```python
from build123d import *

# Parameters (mm, degrees)
SKETCH1_R           = 19.05
BOSS_EXTRUDE1_DEPTH = 1.5875
SKETCH2_R           = 17.4625
BOSS_EXTRUDE2_DEPTH = 12.7
SKETCH3_R           = 7.9375
CUT_EXTRUDE1_DEPTH  = 15.2875
FILLET1_R           = 0.254


with BuildPart() as part:
    # Sketch1 → Boss-Extrude1 (new body)
    with BuildSketch(Plane(origin=(0, 0, 0), x_dir=(1, 0, 0), z_dir=(0, 1, 0))):
        Circle(SKETCH1_R)
    extrude(amount=BOSS_EXTRUDE1_DEPTH)

    # Sketch2 → Boss-Extrude2 (add)
    with BuildSketch(Plane(origin=(0, 1.5875, 0), x_dir=(1, 0, 0), z_dir=(0, 1, 0))):
        Circle(SKETCH2_R)
    extrude(amount=BOSS_EXTRUDE2_DEPTH)

    # Sketch3 → Cut-Extrude1 (cut, through all)
    with BuildSketch(Plane(origin=(0, 14.2875, 0), x_dir=(1, 0, 0), z_dir=(0, 1, 0))):
        Circle(SKETCH3_R)
    extrude(amount=-CUT_EXTRUDE1_DEPTH, mode=Mode.SUBTRACT)

    # Fillet1
    fillet1_edges = [part.edges().sort_by_distance(p)[0] for p in [
        (-7.9375, 14.2875, 0),
        (-19.05, 0, 0),
        (-19.05, 1.5875, 0),
        (-17.4625, 14.2875, 0),
    ]]
    fillet(fillet1_edges, radius=FILLET1_R)


solid = part.part
```
The model under review builds one solid part; all positions refer to its coordinate system, in mm. A direction names the side the tool comes from. Round coordinates to 2 decimals unless told otherwise and drop trailing zeros. Loops run counter-clockwise (first coordinate to the right, second up) from the corner with the lowest first, then second, coordinate; pieces in that order, holes last. Notation, with made-up numbers: M 9.5,33.25 L 43.5,33.25 A19 ccw 43.5,69.25 Z; hole C 5,38 d8. An arc over 180 degrees is marked long. Answer as a JSON object with one key per item and string values.
(1) To check wall thickness, follow line 1 along Z through (x, y) = (0, 8.75); line 2 along X through (y, z) = (6.75, -6.5). State the ranges of each line that lie inside material, in increasing order.
Resolved:
{"line 1": "-17.46 to -7.94, 7.94 to 17.46", "line 2": "-16.21 to -4.56, 4.56 to 16.21"}
(2) Take a section at C-C on y = 10.5. Give the boundary of the cut face in (x, z) (1 decimal), and give its area (3 significant figures).
Resolved:
{"outline": "C 0,0 d34.9; hole C 0,0 d15.9", "area": "760 mm²"}
(3) Draft analysis for pull direction Z (two halves, no side actions). For faces 1 (the flat face through (8.1, 0, -0.3)), 2 (the cylindrical face through (-15.12, 0.79, 11.59)), 3 (the cylindrical face through (-1.72, 7.11, 7.75)), state which applies: released by +Z, released by -Z, zero draft, split by the parting line, or undercut.
Resolved:
{"face 1": "zero draft", "face 2": "split by the parting line", "face 3": "undercut"}
(4) Take a section at A-A on x = 0. Give the boundary of the cut face in (y, z).
Resolved:
{"outline": "M 0,-18.8 A0.25 ccw 0.25,-19.05 L 1.33,-19.05 A0.25 ccw 1.59,-18.8 L 1.59,-17.46 L 14.03,-17.46 A0.25 ccw 14.29,-17.21 L 14.29,-8.19 A0.25 ccw 14.03,-7.94 L 0,-7.94 Z; M 0,7.94 L 14.03,7.94 A0.25 ccw 14.29,8.19 L 14.29,17.21 A0.25 ccw 14.03,17.46 L 1.59,17.46 L 1.59,18.8 A0.25 ccw 1.33,19.05 L 0.25,19.05 A0.25 ccw 0,18.8 Z"}
(5) Tool access review of faces 4 (the flat face through (7.4, 14.288, -4.1)), 5 (the flat face through (5, 1.588, 17)): name each direction out of +Z, -Z, +X, -X, +Y, -Y from which nothing blocks a thin tool from reaching the whole face with its end or side.
Resolved:
{"face 4": "+Z, -Z, +X, -X, +Y", "face 5": "+Y"}
(6) Take a section at B-B on z = 0. Give the boundary of the cut face in (x, y), and give its area (3 significant figures).
Resolved:
{"outline": "M -19.05,0.25 A0.25 ccw -18.8,0 L -7.94,0 L -7.94,14.03 A0.25 ccw -8.19,14.29 L -17.21,14.29 A0.25 ccw -17.46,14.03 L -17.46,1.59 L -18.8,1.59 A0.25 ccw -19.05,1.33 Z; M 7.94,0 L 18.8,0 A0.25 ccw 19.05,0.25 L 19.05,1.33 A0.25 ccw 18.8,1.59 L 17.46,1.59 L 17.46,14.03 A0.25 ccw 17.21,14.29 L 8.19,14.29 A0.25 ccw 7.94,14.03 Z", "area": "277 mm²"}
(7) Clearance check with flat-ended pins moving along their axes: P1, Ø1, axis at x = 4.5, y = 7, coming from the -Z side; P2, Ø4, axis at x = 7.5, y = 8, coming from the +Z side; P3, Ø4, axis at x = 0.5, y = 5, coming from the +Z side; P4, Ø14.5, axis at x = 0, z = 0, coming from the -Y side. State where each tip first meets the part, or that it passes through.
Resolved:
{"P1": "z = -17", "P2": "z = 16.57", "P3": "z = 17.46", "P4": "through"}
